```python
from build123d import *

# Parameters (mm, degrees)
SKIZZE1_W                       = 18
SKIZZE1_H                       = 34.9
SKIZZE1_W_2                     = 14
SKIZZE1_H_2                     = 1.7
AUFSATZ_LINEAR_AUSTRAGEN1_DEPTH = 0.825
VERRUNDUNG1_R                   = 0.8


with BuildPart() as part:
    # Skizze1 → Aufsatz-Linear austragen1 (new body, symmetric)
    with BuildSketch(Plane(origin=(0, 0, 0), x_dir=(1, 0, 0), z_dir=(0, 1, 0))):
        Rectangle(SKIZZE1_W, SKIZZE1_H)
        with Locations((0, 12.4)):
            Rectangle(SKIZZE1_W_2, SKIZZE1_H_2, mode=Mode.SUBTRACT)
        with BuildLine():
            Line((-6, 16.25), (6, 16.25))
            ThreePointArc((6, 16.25), (7.05, 15.2), (6, 14.15))
            Line((6, 14.15), (-6, 14.15))
            ThreePointArc((-6, 14.15), (-7.05, 15.2), (-6, 16.25))
        make_face(mode=Mode.SUBTRACT)
        with BuildLine():
            Line((-6, -16.25), (6, -16.25))
            ThreePointArc((6, -16.25), (7.05, -15.2), (6, -14.15))
            Line((6, -14.15), (-6, -14.15))
            ThreePointArc((-6, -14.15), (-7.05, -15.2), (-6, -16.25))
        make_face(mode=Mode.SUBTRACT)
        with Locations((0, -12.4)):
            Rectangle(SKIZZE1_W_2, SKIZZE1_H_2, mode=Mode.SUBTRACT)
    extrude(amount=AUFSATZ_LINEAR_AUSTRAGEN1_DEPTH, both=True)

    # Verrundung1
    verrundung1_edges = [part.edges().sort_by_distance(p)[0] for p in [
        (-7, 0, -11.55),
        (-7, 0, -13.25),
        (7, 0, -13.25),
        (7, 0, -11.55),
        (7, 0, 13.25),
        (-7, 0, 13.25),
        (-7, 0, 11.55),
        (7, 0, 11.55),
    ]]
    fillet(verrundung1_edges, radius=VERRUNDUNG1_R)


solid = part.part
```
Part model, mm, in its own coordinate system. A direction names the side the tool comes from. Coordinates: 2 decimals unless noted, no trailing zeros. Order: outer loops, then holes, each group sorted by start corner. A loop starts at its lowest first (then second) coordinate and runs counter-clockwise, first axis right, second up. Notation, with made-up numbers: (51.5, -33) - (79.5, -33) arc R9 cw to (79.5, -28) - close; hole circle Ø7 at (37, -37.5). An arc over 180 degrees is marked (long way). Return JSON: item names as keys, results as strings. Group by question number.
Item 1: Cut at D-D (z = 15.5). List the corners of the cut face in (x, y) (3 decimals), plus the area to 3 significant figures.
Item 2: Pull direction X, two halves, no side cores. Call faces 1 (the face through (6.77, -0.01, 13.01)), 2 (the face through (0, 0.825, 0)), 3 (the face through (-9, 0, 0)): pulls with the +X half, pulls with the -X half, needs draft (parallel to the pull), parting line crosses it, or undercut.
Item 3: Cut at C-C (y = 0.2). List the corners of the cut face in (x, z), plus the area to 3 significant figures.
Item 4: Drill centre lines: probe 1 along Z at (x, y) = (4.25, 0.2); probe 2 along Z at (x, y) = (6.75, -0.55); probe 3 along X at (y, z) = (0.75, -15). Where is each one in solid material? Low to high. Write a range as from..to.
Item 5: Which spindle directions (+Z, -Z, +X, -X, +Y, -Y) get a long thin tool onto all of the face, cutting with end or side? Do faces 4 (the face through (9, 0, 0)), 5 (the face through (6.76, -0.01, 11.78)). Say none if no direction does.
Item 6: Cut at B-B (z = -15.2). List the corners of the cut face in (x, y) (3 decimals), plus the area to 4 significant figures.
Item 7: Cut at A-A (x = -4.75). List the corners of the cut face in (y, z) (3 decimals).
Check values:
{
 "1": {"outline": "(-9, -0.825) - (-7.006, -0.825) - (-7.006, 0.825) - (-9, 0.825) - close; (7.006, -0.825) - (9, -0.825) - (9, 0.825) - (7.006, 0.825) - close", "area": "6.58 mm2"},
 "2": {"face 1": "undercut", "face 2": "needs draft", "face 3": "pulls with the -X half"},
 "3": {"outline": "(-9, -17.45) - (9, -17.45) - (9, 17.45) - (-9, 17.45) - close; hole (-7, -12.45) arc R0.8 ccw to (-6.2, -13.25) - (6.2, -13.25) arc R0.8 ccw to (7, -12.45) - (7, -12.35) arc R0.8 ccw to (6.2, -11.55) - (-6.2, -11.55) arc R0.8 ccw to (-7, -12.35) - close; hole (-7, 12.35) arc R0.8 ccw to (-6.2, 11.55) - (6.2, 11.55) arc R0.8 ccw to (7, 12.35) - (7, 12.45) arc R0.8 ccw to (6.2, 13.25) - (-6.2, 13.25) arc R0.8 ccw to (-7, 12.45) - close; hole (-6, -16.25) - (6, -16.25) arc R1.05 ccw to (6, -14.15) - (-6, -14.15) arc R1.05 ccw to start; hole (-6, 14.15) - (6, 14.15) arc R1.05 ccw to (6, 16.25) - (-6, 16.25) arc R1.05 ccw to start", "area": "524 mm2"},
 "4": {"probe 1": "z = -17.45..-16.25, -14.15..-13.25, -11.55..11.55, 13.25..14.15, 16.25..17.45", "probe 2": "z = -17.45..-15.93, -14.47..-13.03, -11.77..11.77, 13.03..14.47, 15.93..17.45", "probe 3": "x = -9..-7.03, 7.03..9"},
 "5": {"face 4": "+Z, -Z, +X, +Y, -Y", "face 5": "+Y, -Y"},
 "6": {"outline": "(-9, -0.825) - (-7.05, -0.825) - (-7.05, 0.825) - (-9, 0.825) - close; (7.05, -0.825) - (9, -0.825) - (9, 0.825) - (7.05, 0.825) - close", "area": "6.435 mm2"},
 "7": {"outline": "(-0.825, -17.45) - (0.825, -17.45) - (0.825, -16.25) - (-0.825, -16.25) - close; (-0.825, -14.15) - (0.825, -14.15) - (0.825, -13.25) - (-0.825, -13.25) - close; (-0.825, -11.55) - (0.825, -11.55) - (0.825, 11.55) - (-0.825, 11.55) - close; (-0.825, 13.25) - (0.825, 13.25) - (0.825, 14.15) - (-0.825, 14.15) - close; (-0.825, 16.25) - (0.825, 16.25) - (0.825, 17.45) - (-0.825, 17.45) - close"}
}
